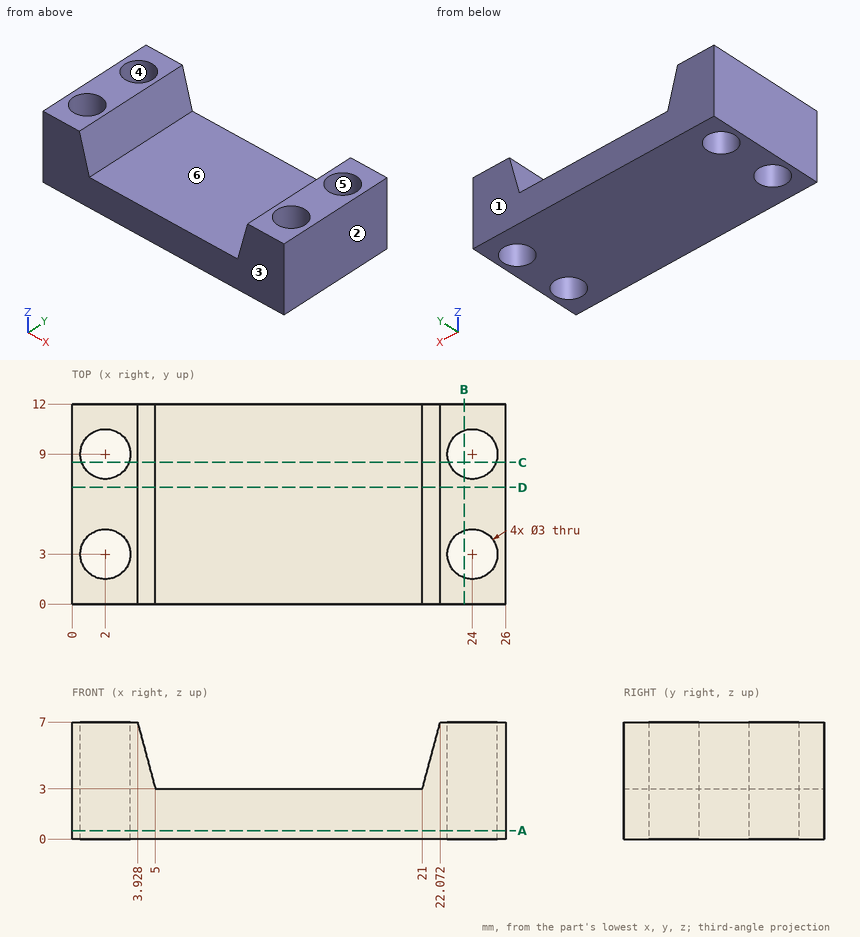
Can you work these out from the drawing? Everything is in mm from the part's minimum corner. A direction names the side the tool comes from. Coordinates: 2 decimals unless noted, no trailing zeros. Loops run counter-clockwise (first coordinate to the right, second up) from the corner with the lowest first, then second, coordinate; pieces in that order, holes last. Notation, with made-up numbers: (75, 48) -> (126, 48) arc R11 ccw to (126, 62) -> close; hole circle Ø5 at (-23, 19.5). An arc over 180 degrees is marked (long way). Return JSON: item names as keys, results as strings.
1) Thinking about a two-plate mould opening in Y: for the marked faces 1, 2, 3 and 4, which applies, +Y half, -Y half, draft (parallel to the pull), parting line (faces both ways), or undercut?
Results below:
{"face 1": "+Y half", "face 2": "draft", "face 3": "-Y half", "face 4": "undercut"}
2) If we section it at A-A, the plane z = 0.5: Write out the boundary of the cut face in (x, y).
Results below:
{"outline": "(0, 0) -> (26, 0) -> (26, 12) -> (0, 12) -> close; hole circle Ø3 at (2, 3); hole circle Ø3 at (2, 9); hole circle Ø3 at (24, 3); hole circle Ø3 at (24, 9)"}
3) For the marked faces 5 and 6, which set-ups out of +Z, -Z, +X, -X, +Y, -Y let a thin tool reach every point of the face, with its end or its side?
Results below:
{"face 5": "+Z, -Z", "face 6": "+Z, +Y, -Y"}
4) If we section it at C-C, the plane y = 8.5: Write out the boundary of the cut face in (x, z).
Results below:
{"outline": "(0, 0) -> (0.59, 0) -> (0.59, 7) -> (0, 7) -> close; (3.41, 0) -> (22.59, 0) -> (22.59, 7) -> (22.07, 7) -> (21, 3) -> (5, 3) -> (3.93, 7) -> (3.41, 7) -> close; (25.41, 0) -> (26, 0) -> (26, 7) -> (25.41, 7) -> close"}
5) Will this pin go through, and if not, where does the flat tip stop? pin 1 (1 mm diameter, centred on y = 9, z = 2.5, fed in from -X).
Results below:
{"pin 1": "x = 0"}
6) I need wall thicknesses on line 1 (Y direction, x = 24, z = 4); line 2 (X direction, y = 1.75, z = 3.75); line 3 (X direction, y = 8.5, z = 1.25). Which ranges of each line are inside material? Lowest first, please. Write a range as from..to.
Results below:
{"line 1": "0..1.5, 4.5..7.5, 10.5..12", "line 2": "0..1.17, 2.83..4.8, 21.2..23.17, 24.83..26", "line 3": "0..0.59, 3.41..22.59, 25.41..26"}
7) If we section it at B-B, the plane x = 23.5: Write out the boundary of the cut face in (y, z), then the cut area to 3 significant figures.
Results below:
{"outline": "(0, 0) -> (1.59, 0) -> (1.59, 7) -> (0, 7) -> close; (4.41, 0) -> (7.59, 0) -> (7.59, 7) -> (4.41, 7) -> close; (10.41, 0) -> (12, 0) -> (12, 7) -> (10.41, 7) -> close", "area": "44.4 mm²"}
8) If we section it at D-D, the plane y = 7: Write out the boundary of the cut face in (x, z).
Results below:
{"outline": "(0, 0) -> (26, 0) -> (26, 7) -> (22.07, 7) -> (21, 3) -> (5, 3) -> (3.93, 7) -> (0, 7) -> close"}
